Can you work these out from the model? Positions are in its coordinate system, mm. A direction names the side the tool comes from. Round coordinates to 2 decimals unless told otherwise and drop trailing zeros. Loops run counter-clockwise (first coordinate to the right, second up) from the corner with the lowest first, then second, coordinate; pieces in that order, holes last. Notation, with made-up numbers: M 7,25.5 L 54,25.5 A27 ccw 54,48.5 Z; hole C -29,29 d8. An arc over 180 degrees is marked long. Return JSON: item names as keys, results as strings.
```python
from build123d import *

# Parameters (mm, degrees)
F0_W     = 300
F0_H     = 300
F1_DEPTH = 300
F2_T     = -9
F3_W     = 282
F3_H     = 15.1234567165
F3_W_2   = 16.8518549763
F3_H_2   = 10.3703700006
F3_H_3   = 99.3024680614
F4_DEPTH = 288


with BuildPart() as f1:
    # F0 (on Front) → F1 (new body)
    with BuildSketch(Plane.XZ):
        Rectangle(F0_W, F0_H)
    extrude(amount=-F1_DEPTH)

    # F2
    f2_openings = [f1.faces().sort_by_distance(p)[0] for p in [
        (0, 0, 0),
    ]]
    offset(amount=F2_T, openings=f2_openings)

    # F3 (on face) → F4 (join)
    with BuildSketch(Plane.XZ.offset(-291)):
        Polygon((-141, 41.6975319386), (-141, 23.9814817905), (141, 23.9814817905), (141, 41.6975319386), (9.9382726476, 41.6975319386), (9.9382726476, 31.327161938), (-6.9135823287, 31.327161938), (-6.9135823287, 41.6975319386), align=None)
        with Locations((0, -69.1358074546)):
            Rectangle(F3_W, F3_H)
        with Locations((1.5123451594, 36.5123469383)):
            Rectangle(F3_W_2, F3_H_2)
        with Locations((1.5123451594, 91.3487659693)):
            Rectangle(F3_W_2, F3_H_3)
    extrude(amount=F4_DEPTH)


solid = f1.part
```
Q1. Suppose I cut it at C-C, the plane y = 240.5. Please give me the cut outline in (x, z).
Results:
{"outline": "M -150,-150 L 150,-150 L 150,150 L -150,150 Z; hole M -141,-141 L 141,-141 L 141,-76.7 L -141,-76.7 Z; hole M -141,-61.57 L 141,-61.57 L 141,23.98 L -141,23.98 Z; hole M -141,41.7 L -6.91,41.7 L -6.91,141 L -141,141 Z; hole M 9.94,41.7 L 141,41.7 L 141,141 L 9.94,141 Z"}
Q2. If I drill on line 1 along Z through (x, y) = (21, 239.5); line 2 along X through (y, z) = (203, 67.5); line 3 along X through (y, z) = (203, 1), over which ranges is the centre line in solid material (lowest first)?
Results:
{"line 1": "z = -150 to -141, -76.7 to -61.57, 23.98 to 41.7, 141 to 150", "line 2": "x = -150 to -141, -6.91 to 9.94, 141 to 150", "line 3": "x = -150 to -141, 141 to 150"}
Q3. Suppose I cut it at D-D, the plane z = -99. Please give me the cut outline in (x, y).
Results:
{"outline": "M -150,0 L -141,0 L -141,291 L 141,291 L 141,0 L 150,0 L 150,300 L -150,300 Z"}
Q4. Thinking about a two-plate mould opening in X: for faces 3 (the flat face through (141, 143, -2)), 4 (the flat face through (-6.914, 149, 91)), 5 (the flat face through (-150, 148, -2)), 6 (the flat face through (-2, 148, 150)), which applies, pulls with the +X half, pulls with the -X half, needs draft (parallel to the pull), parting line crosses it, or undercut?
Results:
{"face 3": "undercut", "face 4": "undercut", "face 5": "pulls with the -X half", "face 6": "needs draft"}
Q5. Suppose I cut it at B-B, the plane x = -51. Please give me the cut outline in (y, z).
Results:
{"outline": "M 0,-150 L 300,-150 L 300,150 L 0,150 L 0,141 L 291,141 L 291,41.7 L 3,41.7 L 3,23.98 L 291,23.98 L 291,-61.57 L 3,-61.57 L 3,-76.7 L 291,-76.7 L 291,-141 L 0,-141 Z"}
Q6. On a 3-axis mill with a long thin cutter (end or side, diameter ignored), from which of +Z, -Z, +X, -X, +Y, -Y can I reach the whole of each face in a straight line? I mean faces 1 (the flat face through (29, 143, 141)), 2 (the flat face through (-12, 0, -144)). Say none if no direction works.
Results:
{"face 1": "-Y", "face 2": "+Z, -Z, +X, -X, -Y"}
Q7. Suppose I cut it at A-A, the plane z = 71.5. Please give me the cut outline in (x, y).
Results:
{"outline": "M -150,0 L -141,0 L -141,291 L -6.91,291 L -6.91,3 L 9.94,3 L 9.94,291 L 141,291 L 141,0 L 150,0 L 150,300 L -150,300 Z"}
Q8. I'm going to push flat-ended pins straight in: pin 1 Ø4.5 at (x, z) = (22, -67.5) entering from -Y; pin 2 Ø12 at (x, z) = (78, -83) entering from -Y. Where does each tip first touch, or does it pass through?
Results:
{"pin 1": "stops at y = 3", "pin 2": "stops at y = 291"}
